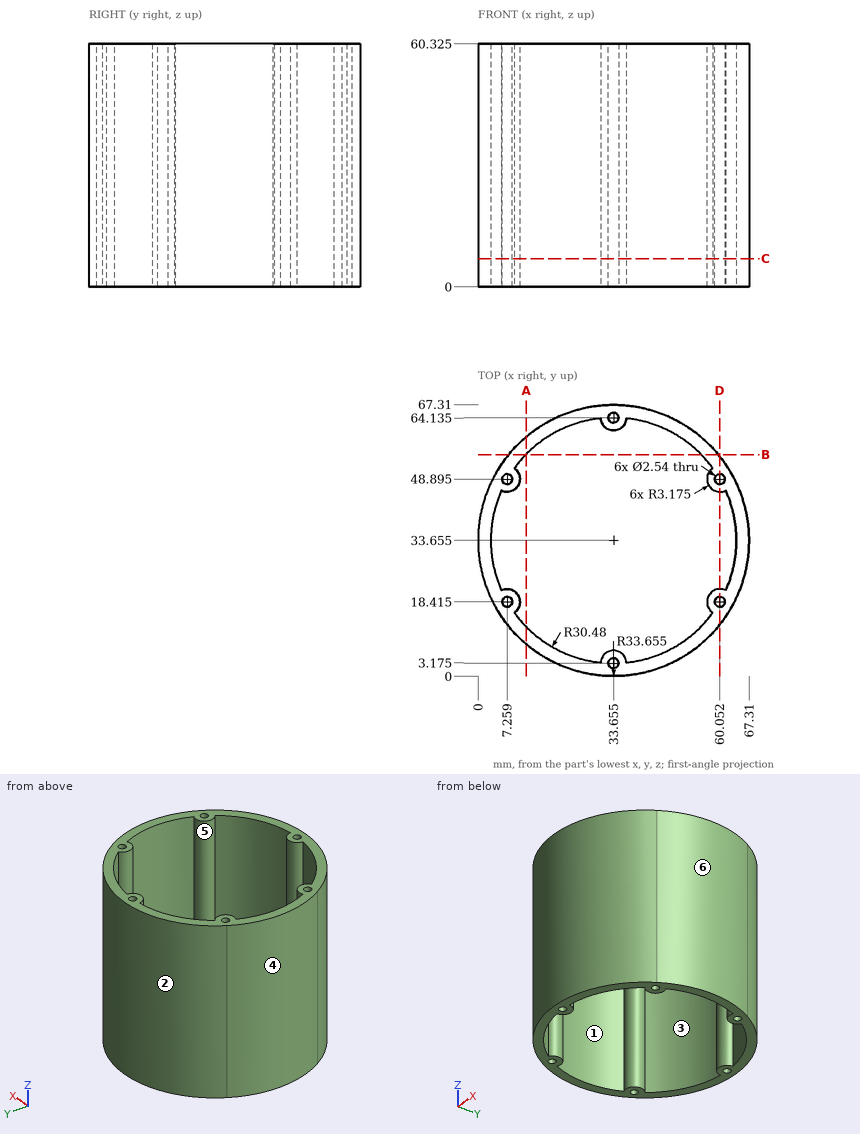
Can you work these out from the drawing? Everything is in mm from the part's minimum corner. A direction names the side the tool comes from. Round coordinates to 2 decimals unless told otherwise and drop trailing zeros. Loops run counter-clockwise (first coordinate to the right, second up) from the corner with the lowest first, then second, coordinate; pieces in that order, holes last. Notation, with made-up numbers: (0, -18) -> (32, -18) arc R18 ccw to (32, -10) -> close; hole circle Ø9 at (-29.75, -12.75). An arc over 180 degrees is marked (long way). Answer in a Markdown table with one row per item.
Item 1: Suppose I cut it at D-D, the plane x = 60. List the corners of the cut face in (y, z) for me (1 decimal).
Answer block:
| item | result |
|---|---|
| outline | (12.7, 0) -> (17.1, 0) -> (17.1, 60.3) -> (12.7, 60.3) -> close; (19.7, 0) -> (21.6, 0) -> (21.6, 60.3) -> (19.7, 60.3) -> close; (45.7, 0) -> (47.6, 0) -> (47.6, 60.3) -> (45.7, 60.3) -> close; (50.2, 0) -> (54.6, 0) -> (54.6, 60.3) -> (50.2, 60.3) -> close |
Item 2: We'd pull the mould along X, two halves only. Please class the marked faces 3, 4, 5 and 6: released by +X, released by -X, zero draft, split by the parting line, or undercut.
Answer block:
| item | result |
|---|---|
| face 3 | undercut |
| face 4 | released by -X |
| face 5 | undercut |
| face 6 | released by +X |
Item 3: Suppose I cut it at C-C, the plane z = 7. Give the number of separate pieces and of enclosed holes in the cut face.
Answer block:
| item | result |
|---|---|
| separate pieces | 1 |
| enclosed holes | 7 |
Item 4: Suppose I cut it at B-B, the plane y = 55. List the corners of the cut face in (x, z) for me (1 decimal).
Answer block:
| item | result |
|---|---|
| outline | (7.6, 0) -> (11.9, 0) -> (11.9, 60.3) -> (7.6, 60.3) -> close; (55.4, 0) -> (59.7, 0) -> (59.7, 60.3) -> (55.4, 60.3) -> close |
Item 5: If I drill on probe 1 along Y at (x, z) = (33.5, 27.5) (1 decimal); probe 2 along Y at (x, z) = (15.5, 39) (1 decimal); probe 3 along X at (y, z) = (22, 40), over which ranges is the centre line in solid material (lowest first)?
Answer block:
| item | result |
|---|---|
| probe 1 | 0 to 1.9, 4.4 to 6.3, 61 to 62.9, 65.4 to 67.3 |
| probe 2 | 5.3 to 9.2, 58.1 to 62 |
| probe 3 | 2.08 to 5.49, 61.82 to 65.23 |
Item 6: Suppose I cut it at A-A, the plane x = 12. List the corners of the cut face in (y, z) for me (1 decimal).
Answer block:
| item | result |
|---|---|
| outline | (7.9, 0) -> (12.2, 0) -> (12.2, 60.3) -> (7.9, 60.3) -> close; (55.1, 0) -> (59.4, 0) -> (59.4, 60.3) -> (55.1, 60.3) -> close |
Item 7: On a 3-axis mill with a long thin cutter (end or side, diameter ignored), from which of +Z, -Z, +X, -X, +Y, -Y can I reach the whole of each face in a straight line? I mean the marked faces 1 and 2. Say none if no direction works.
Answer block:
| item | result |
|---|---|
| face 1 | +Z, -Z |
| face 2 | +Z, -Z, +Y |
Item 8: Will these pins go through, and if not, where does the flat tip stop? P1, Ø12, axis at x = 54.5, z = 24.5, coming from the +Y side; P2, Ø5, axis at x = 15.5, z = 30.5, coming from the +Y side; P3, Ø2, axis at x = 48.5, z = 16.5, coming from the +Y side.
Answer block:
| item | result |
|---|---|
| P1 | y = 63.86 |
| P2 | y = 63.45 |
| P3 | y = 64.33 |
